from build123d import *

# Parameters (mm, degrees)
SKETCH001_R     = 5.5
SKETCH001_R_2   = 3.5
POCKET_DEPTH    = 0.2
SKETCH002_R     = 5.5
SKETCH002_R_2   = 3.5
POCKET001_DEPTH = 0.2


with BuildPart() as part:
    # Sketch → Revolution (revolve)
    with BuildSketch(Plane.XZ):
        Polygon((2.5, 4), (6.5, 4), (6.5, 1), (7.5, 1), (7.5, 0), (2.5, 0), align=None)
    revolve(axis=Axis((0, 0, 0), (0, 0, 1)))

    # Sketch001 (on Face1 of Revolution) → Pocket (cut)
    with BuildSketch(Plane(origin=(0, 0, 4), x_dir=(-1, 0, 0), z_dir=(0, 0, 1))):
        Circle(SKETCH001_R)
        Circle(SKETCH001_R_2, mode=Mode.SUBTRACT)
    extrude(amount=-POCKET_DEPTH, mode=Mode.SUBTRACT)

    # Sketch002 (on Face8 of Pocket) → Pocket001 (cut)
    with BuildSketch(Plane(origin=(0, 0, 0), x_dir=(1, 0, 0), z_dir=(0, 0, -1))):
        Circle(SKETCH002_R)
        Circle(SKETCH002_R_2, mode=Mode.SUBTRACT)
    extrude(amount=-POCKET001_DEPTH, mode=Mode.SUBTRACT)


solid = part.part
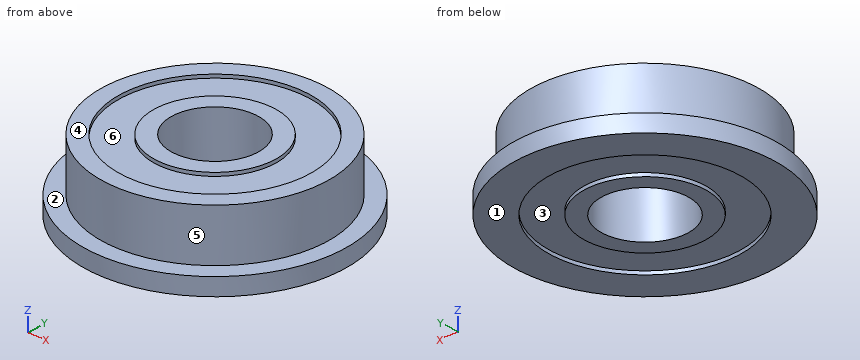
Input: part model. Units: mm. Frame: model coordinates. Face numbers are marked on the shaded views. A direction names the side the tool comes from. Coordinates: 2 decimals unless noted, no trailing zeros. Loops run counter-clockwise (first coordinate to the right, second up) from the corner with the lowest first, then second, coordinate; pieces in that order, holes last.
(1) Section A-A on x = 0. Return the cut outline in (y, z).
(2) Set-up query: the marked faces 1, 2 and 3. Return all of +Z, -Z, +X, -X, +Y, -Y with unobstructed straight access to the full face (end or side cutting, diameter ignored); none if empty.
(3) First-contact query: pin 1 Ø1.5 at (y, z) = (5, 3.5) entering from -X; pin 2 Ø1.5 at (x, z) = (2.5, 0.5) entering from +Y. Flat tips, straight axial feed; report the tip coordinate or a pass-through.
(4) Section C-C on z = 0.65. Return the cut outline in (x, y).
(5) Section D-D on x = 3.25. Return the cut outline in (y, z).
(6) Pull-direction query (Y, two-part tool) for the marked faces 4, 5 and 6; classes: released by +Y, released by -Y, zero draft, split by the parting line, or undercut.
(7) Material intervals for probe 1 along Y at (x, z) = (0, 0.1); probe 2 along Y at (x, z) = (0, 0.8); probe 3 along Z at (x, y) = (3.75, 1.25), sorted ascending.
Data:
1. outline: (-7.5, 0) - (-5.5, 0) - (-5.5, 0.2) - (-3.5, 0.2) - (-3.5, 0) - (-2.5, 0) - (-2.5, 4) - (-3.5, 4) - (-3.5, 3.8) - (-5.5, 3.8) - (-5.5, 4) - (-6.5, 4) - (-6.5, 1) - (-7.5, 1) - close; (2.5, 0) - (3.5, 0) - (3.5, 0.2) - (5.5, 0.2) - (5.5, 0) - (7.5, 0) - (7.5, 1) - (6.5, 1) - (6.5, 4) - (5.5, 4) - (5.5, 3.8) - (3.5, 3.8) - (3.5, 4) - (2.5, 4) - close
2. face 1: -Z, +X, -X, +Y, -Y
2. face 2: +Z
2. face 3: -Z
3. pin 1: stops at x = -4.92
3. pin 2: stops at y = 7.29
4. outline: circle Ø15 at (0, 0); hole circle Ø5 at (0, 0)
5. outline: (-6.76, 0) - (-4.44, 0) - (-4.44, 0.2) - (-1.3, 0.2) - (-1.3, 0) - (1.3, 0) - (1.3, 0.2) - (4.44, 0.2) - (4.44, 0) - (6.76, 0) - (6.76, 1) - (5.63, 1) - (5.63, 4) - (4.44, 4) - (4.44, 3.8) - (1.3, 3.8) - (1.3, 4) - (-1.3, 4) - (-1.3, 3.8) - (-4.44, 3.8) - (-4.44, 4) - (-5.63, 4) - (-5.63, 1) - (-6.76, 1) - close
6. face 4: zero draft
6. face 5: split by the parting line
6. face 6: undercut
7. probe 1: y = -7.5 to -5.5, -3.5 to -2.5, 2.5 to 3.5, 5.5 to 7.5
7. probe 2: y = -7.5 to -2.5, 2.5 to 7.5
7. probe 3: z = 0.2 to 3.8
